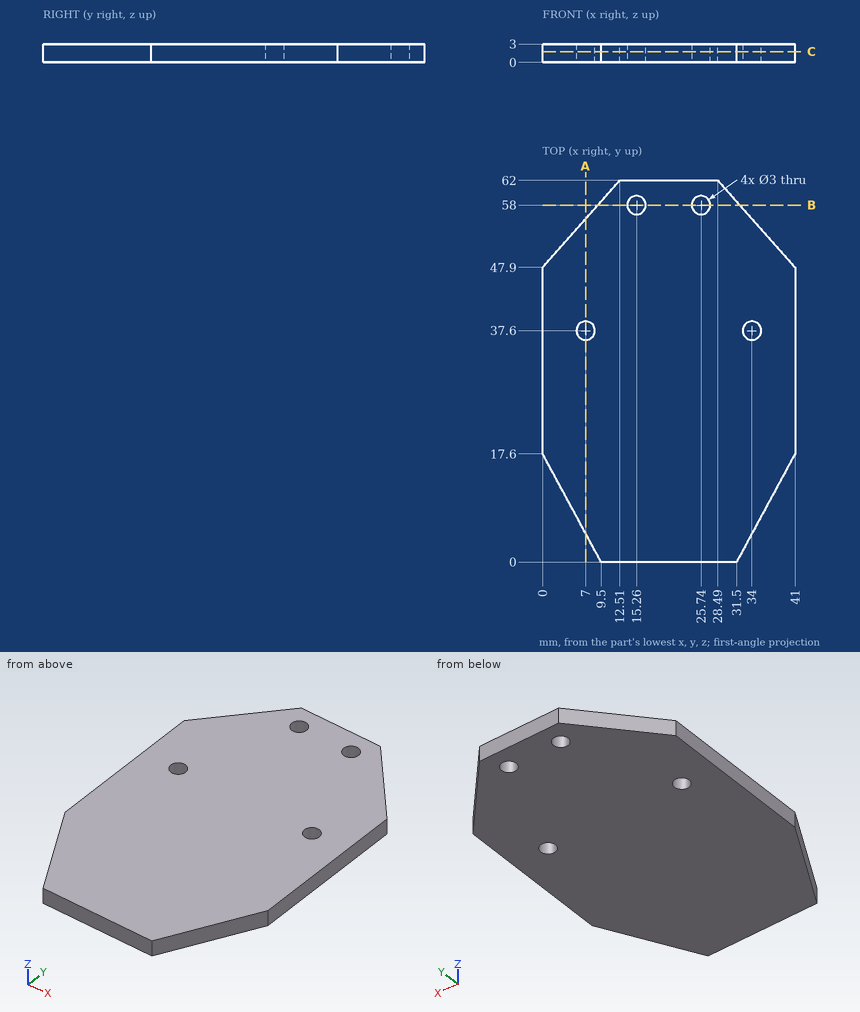
Input: dimensioned drawing with shaded views. Units: mm. Origin: part minimum x, y, z. Give positions to 0.01 mm unless a question says otherwise; leave off trailing zeros. Write each loop counter-clockwise with the first axis right and the second up, starting at its lowest first coordinate (ties: lowest second). Pieces come first, ordered by that corner, then holes.
1. Section query B-B (y = 58). Return the cut outline in (x, z).
2. Section query A-A (x = 7). Return the cut outline in (y, z).
3. Section query C-C (z = 1.75). Return the cut outline in (x, y), then the cut area to 3 significant figures.
4. First-contact query: pin 1 (1.8 mm diameter, centred on x = 34, y = 37.6, fed in from +Z) (3 decimals). Flat tip, straight axial feed; report the tip coordinate or a pass-through.
5. Material intervals for line 1 along Y through (x, z) = (7.5, 2.1) (1 decimal); line 2 along Y through (x, z) = (7, 1.2); line 3 along X through (y, z) = (3, 2.25), sorted ascending.
Output values:
1. outline: (8.96, 0) - (13.76, 0) - (13.76, 3) - (8.96, 3) - close; (16.76, 0) - (24.24, 0) - (24.24, 3) - (16.76, 3) - close; (27.24, 0) - (32.04, 0) - (32.04, 3) - (27.24, 3) - close
2. outline: (4.63, 0) - (36.1, 0) - (36.1, 3) - (4.63, 3) - close; (39.1, 0) - (55.79, 0) - (55.79, 3) - (39.1, 3) - close
3. outline: (0, 17.6) - (9.5, 0) - (31.5, 0) - (41, 17.6) - (41, 47.9) - (28.49, 62) - (12.51, 62) - (0, 47.9) - close; hole circle Ø3 at (7, 37.6); hole circle Ø3 at (15.26, 58); hole circle Ø3 at (25.74, 58); hole circle Ø3 at (34, 37.6)
3. area: 2,170 mm2
4. pin 1: passes through
5. line 1: y = 3.7 to 36.2, 39 to 56.4
5. line 2: y = 4.63 to 36.1, 39.1 to 55.79
5. line 3: x = 7.88 to 33.12
